Autodesk Inventor part; units mm, degrees
ref_plane "YZ Plane" through (0, 0, 0) normal (1, 0, 0) x (0, 1, 0)
ref_plane "XZ Plane" through (0, 0, 0) normal (0, 1, 0) x (-1, 0, 0)
ref_plane "XY Plane" through (0, 0, 0) normal (0, 0, 1) x (1, 0, 0)
sketch "スケッチ1" plane through (0, 0, 0) normal (0, 1, 0) x (-1, 0, 0)
  line L0 (8.5, 15.5) -> (-8.5, 15.5) construction
  line L1 (-8.5, 15.5) -> (-8.5, -15.5)
  line L2 (-8.5, -15.5) -> (8.5, -15.5) construction
  line L3 (8.5, -15.5) -> (8.5, 15.5)
  circle A0 centre (0, 8.5) radius 7
  circle A1 centre (0, -8.5) radius 7
  circle A2 centre (6.75, -13.5) radius 0.8
  line L4 (6.75, -13.5) -> (-6.75, -13.5) construction
  line L5 (-6.75, -13.5) -> (-6.75, 13.5) construction
  line L6 (-6.75, 13.5) -> (6.75, 13.5) construction
  line L7 (6.75, 13.5) -> (6.75, -13.5) construction
  circle A3 centre (-6.75, -13.5) radius 0.8
  circle A4 centre (6.75, 13.5) radius 0.8
  circle A5 centre (-6.75, 13.5) radius 0.8
  line L8 (8.5, 18.5) -> (-8.5, 18.5)
  line L9 (-8.5, 18.5) -> (-8.5, 15.5)
  line L10 (-8.5, 15.5) -> (8.5, 15.5)
  line L11 (8.5, 15.5) -> (8.5, 18.5)
  line L12 (8.5, -15.5) -> (-8.5, -15.5)
  line L13 (-8.5, -15.5) -> (-8.5, -18.5)
  line L14 (-8.5, -18.5) -> (8.5, -18.5)
  line L15 (8.5, -18.5) -> (8.5, -15.5)
  line L16 (-6.75, 10.354) -> (-6.75, -10.354)
  line L17 (13.5, -1.5) -> (-13.5, -1.5)
  line L18 (-13.5, -1.5) -> (-13.5, 1.5)
  line L19 (-13.5, 1.5) -> (13.5, 1.5)
  line L20 (13.5, 1.5) -> (13.5, -1.5)
  point P0 (0, 0)
  point P1 (0, 0)
  point P2 (0, 15.5)
  point P3 (8.5, 0)
  point P4 (6.75, 0)
  point P5 (0, 13.5)
  point P6 (6.75, 10.354)
  point P7 (6.75, -10.354)
  point P8 (7, 8.5)
  point P9 (7, -8.5)
  point P10 (-7, 8.5)
  point P11 (-7, -8.5)
  point P12 (-6.75, -6.646)
  point P13 (-6.75, 6.646)
  point P14 (13.5, 0)
  point P15 (0, -1.5)
  point P16 (8.5, 1.5)
  point P17 (8.5, -1.5)
  point P18 (-8.5, -1.5)
  point P19 (-8.5, 1.5)
  dimension "d0" = 17
  dimension "d1" = 31
  dimension "d2" = 14
  dimension "d4" = 27
  dimension "d5" = 13.5
  dimension "d7" = 1.6
  dimension "d9" = 3
  dimension "d26" = 5
extrude "押し出し1" add sketch "スケッチ1" against normal blind 3 contours L10 A0 L16 L19 L1 | L9 L8 L11 L10 | L19 L16 L17 L1 | L1 L17 L18 L19 | L10 L3 L19 A0 | L17 L16 A1 L12 L1 | L19 L3 L17 L16 | L16 A0 L19 | L12 L15 L14 L13 | L17 A1 L16 | L19 L20 L17 L3 | A1 L17 L3 L12
extrude "押し出し2" add sketch "スケッチ1" along normal blind 1.6 contours L9 L8 L11 L10 | L12 L15 L14 L13
sketch "スケッチ4" plane through (0, -3, 0) normal (0, -1, 0) x (1, 0, 0)
  line L0 (-8.5, 1.5) -> (-13.5, 1.5)
  line L1 (-13.5, 1.5) -> (-13.5, -1.5)
  line L2 (-13.5, -1.5) -> (-8.5, -1.5)
  line L3 (8.5, -1.5) -> (13.5, -1.5)
  line L4 (13.5, -1.5) -> (13.5, 1.5)
  line L5 (13.5, 1.5) -> (8.5, 1.5)
  line L6 (-13.5, -1.5) -> (13.5, -1.5)
  line L7 (-8.5, 1.5) -> (-13.5, 1.5)
  line L8 (-13.5, 1.5) -> (13.5, 1.5)
  line L9 (13.5, 1.5) -> (13.5, -1.5)
  line L10 (13.5, -1.5) -> (-13.5, -1.5)
  line L11 (-13.5, -1.5) -> (-13.5, 1.5)
  point P0 (-7, -1.5)
  point P1 (7, -1.5)
  point P2 (7, 1.5)
  point P3 (-7, 1.5)
  point P4 (0, 0)
  point P5 (-8.5, -1.5)
  point P6 (7, -1.5)
  point P7 (8.5, -1.5)
  point P8 (8.5, 1.5)
  point P9 (-7, 1.5)
extrude "押し出し4" add sketch "スケッチ4" along normal blind 2
sketch "スケッチ2" plane through (-8.5, -3, 18.5) normal (0, 0, 1) x (1, 0, 0)
  line L0 (0, 4.6) -> (17, 4.6)
  circle A0 centre (8.5, 13) radius 2.5
  line L1 (17, 4.6) -> (0, 4.6)
  line L2 (0, 4.6) -> (6.4096, 14.3712)
  line L3 (17, 4.6) -> (10.5904, 14.3712)
  point P0 (8.5, 3)
  dimension "d14" = 10
  dimension "d15" = 5
extrude "押し出し3" add sketch "スケッチ2" against normal up to surface (3 mm away)
sketch "スケッチ3" plane through (-8.5, -3, 18.5) normal (0, 0, 1) x (1, 0, 0)
  arc A0 (10.5904, 14.3712) -> (6.4096, 14.3712) centre (8.5, 13) ccw
  point P0 (8.5, 3)
hole "穴1" at (0, 10, 18.5) direction (0, 0, -1) diameter 2.2 end through all
properties part number "Ultrasonic_holderV3"
Here's how the part is built. I have some questions about the finished solid (model axes, mm). A direction names the side the tool comes from. Give positions to 0.01 mm unless a question says otherwise; leave off trailing zeros. Order: outer loops, then holes, each group sorted by start corner. A loop starts at its lowest first (then second) coordinate and runs counter-clockwise, first axis right, second up. Notation, with made-up numbers: M 66,-14 L 100,-14 A13 ccw 100,5 Z; hole C 83.5,3.25 d9. An arc over 180 degrees is marked long. Use a Markdown table: item, result. Add a question column.
1. Suppose I cut it at A-A (y = 0.5). List the corners of the cut face in (x, z) for me, and give its area (3 significant figures).
2. Suppose I cut it at C-C (x = -5.5). List the corners of the cut face in (y, z) for me, and give its area (3 significant figures).
3. Suppose I cut it at D-D (y = -1.75). List the corners of the cut face in (x, z) for me, and give its area (3 significant figures).
4. Suppose I cut it at B-B (z = -8.5). List the corners of the cut face in (x, y) for me.
5. For pin 1 Ø5 at (y, z) = (-1, -11.5) entering from -X; pin 2 Ø2.5 at (x, z) = (6.75, 13.5) entering from -Y; pin 3 Ø1.4 at (y, z) = (-1, -7) entering from +X, each with a flat end and sliding along its axis, tell me the tip position at first contact or that it passes through.
6. I need wall thicknesses on probe 1 along Z at (x, y) = (0, -2.3); probe 2 along Z at (x, y) = (2, 1); probe 3 along Z at (x, y) = (3.75, -1.5). Which ranges of each line are inside material? Lowest first, please. Write a range as from..to.
7. On a 3-axis mill with a long thin cutter (end or side, diameter ignored), from which of +Z, -Z, +X, -X, +Y, -Y can I reach the whole of each face in a straight line? I mean faces 5 (the flat face through (8.5, -1, 10)), 6 (the flat face through (0, 5, 15.5)), 7 (the flat face through (0, -3, -16)). Say none if no direction works.
8. If we mould it in two halves opening along Z, with no side actions, what happens to faces 1 (the cylindrical face through (-6.16, -1.48, 14.04)), 2 (the flat face through (-5.34, 6.42, 17.02)), 3 (the cylindrical face through (7.34, -1.48, 14.04)), 4 (the flat face through (0, -1, -18.5))? For each: +Z half, -Z half, draft (parallel to the pull), parting line (faces both ways), or undercut.
Results list:
| question | item | result |
|---|---|---|
| 1 | outline | M -8.5,-18.5 L 8.5,-18.5 L 8.5,-15.5 L -8.5,-15.5 Z; M -8.5,15.5 L 8.5,15.5 L 8.5,18.5 L -8.5,18.5 Z |
| 1 | area | 102 mm² |
| 2 | outline | M -5,-1.5 L -3,-1.5 L -3,-4.17 L 0,-4.17 L 0,4.17 L -3,4.17 L -3,1.5 L -5,1.5 Z; M -3,-18.5 L 1.6,-18.5 L 1.6,-15.5 L 0,-15.5 L 0,-12.83 L -3,-12.83 Z; M -3,12.83 L 0,12.83 L 0,15.5 L 6.17,15.5 L 6.17,18.5 L -3,18.5 Z |
| 2 | area | 88.4 mm² |
| 3 | outline | M -13.5,-1.5 L -8.5,-1.5 L -8.5,-18.5 L 8.5,-18.5 L 8.5,-1.5 L 13.5,-1.5 L 13.5,1.5 L 8.5,1.5 L 8.5,18.5 L -8.5,18.5 L -8.5,1.5 L -13.5,1.5 Z; hole C -6.75,-13.5 d1.6; hole C -6.75,13.5 d1.6; hole C 0,-8.5 d14; hole C 0,8.5 d14; hole C 6.75,-13.5 d1.6; hole C 6.75,13.5 d1.6 |
| 3 | area | 343 mm² |
| 4 | outline | M -8.5,-3 L -7,-3 L -7,0 L -8.5,0 Z; M 7,-3 L 8.5,-3 L 8.5,0 L 7,0 Z |
| 5 | pin 1 | stops at x = -8.5 |
| 5 | pin 2 | stops at y = -3 |
| 5 | pin 3 | stops at x = 8.5 |
| 6 | probe 1 | z = -18.5..-15.5, -1.5..1.5, 15.5..18.5 |
| 6 | probe 2 | z = -18.5..-15.5, 15.5..18.5 |
| 6 | probe 3 | z = -18.5..-14.41, -2.59..2.59, 14.41..18.5 |
| 7 | face 5 | +Z, +X, +Y, -Y |
| 7 | face 6 | +X, -X, +Y |
| 7 | face 7 | -Z, +X, -X, -Y |
| 8 | face 1 | undercut |
| 8 | face 2 | draft |
| 8 | face 3 | undercut |
| 8 | face 4 | -Z half |
